```python
from build123d import *

# Parameters (mm, degrees)
SKETCH1_W           = 12.7
SKETCH1_H           = 9.525
BOSS_EXTRUDE1_DEPTH = 2.54
FILLET1_R           = 0.635
SHELL1_START        = 0.635
SHELL1_OUTLINE_W    = 1.905
SHELL1_OUTLINE_H    = 8.255
SHELL1_DEPTH        = 11.43
SKETCH2_R           = 2.54
BOSS_EXTRUDE2_DEPTH = 1.905
BOSS_EXTRUDE3_DEPTH = 0.00254


# Read off the part's stored shape, not the designer's step: Shell1
with BuildPart() as part:
    # Sketch1 → Boss-Extrude1 (new body)
    with BuildSketch(Plane(origin=(0, 0, 0), x_dir=(1, 0, 0), z_dir=(0, 1, 0))):
        with Locations((6.35, 4.7625)):
            Rectangle(SKETCH1_W, SKETCH1_H)
    extrude(amount=BOSS_EXTRUDE1_DEPTH)

    # Fillet1
    fillet1_edges = [part.edges().sort_by_distance(p)[0] for p in [
        (0, 1.27, -9.525),
        (12.7, 1.27, -9.525),
        (12.7, 1.27, 0),
        (0, 1.27, 0),
    ]]
    fillet(fillet1_edges, radius=FILLET1_R)

    # Shell1 outline → Shell1 (cut)
    with BuildSketch(Plane.YZ.offset(SHELL1_START)):
        with Locations((0.9525, -4.7625)):
            Rectangle(SHELL1_OUTLINE_W, SHELL1_OUTLINE_H)
    extrude(amount=SHELL1_DEPTH, mode=Mode.SUBTRACT)

    # Sketch2 → Boss-Extrude2 (add)
    with BuildSketch(Plane(origin=(0, 1.905, 0), x_dir=(-1, 0, 0), z_dir=(0, -1, 0))):
        with Locations(Location((-6.35, 4.7625, 0), (0, 0, 270))):
            Circle(SKETCH2_R)
    extrude(amount=BOSS_EXTRUDE2_DEPTH)

    # Sketch3 → Boss-Extrude3 (add)
    with BuildSketch(Plane(origin=(0, 2.54, 0), x_dir=(1, 0, 0), z_dir=(0, 1, 0))):
        Polygon((4.557346154, 6.477), (6.104141026, 6.477), (6.104141026, 5.907128205), (5.127217949, 5.907128205), (5.127217949, 5.296551282), (6.104141026, 5.296551282), (6.104141026, 4.726679487), (5.127217949, 4.726679487), (5.127217949, 3.302), (4.557346154, 3.302), align=None)
        with BuildLine():
            Line((7.162474359, 5.703602564), (6.592602564, 5.703602564))
            add(Edge.make_bspline(
                [(6.592602564, 5.703602564), (6.596626076, 5.732088422), (6.604513904, 5.78793306), (6.623388421, 5.868782184), (6.645964381, 5.945473111), (6.674149313, 6.017762976), (6.707205653, 6.085780553), (6.744797255, 6.149759244), (6.787330498, 6.20942444), (6.81993268, 6.245366991), (6.836197316, 6.263298077)],
                knots=[0, 0, 0, 0, 1.111473889, 2.178970933, 3.205615836, 4.199322666, 5.174200091, 6.12565194, 7.064921805, 8, 8, 8, 8], degree=3))
            add(Edge.make_bspline(
                [(6.836197316, 6.263298077), (6.859656898, 6.286956845), (6.905893269, 6.333585791), (6.983159668, 6.39331232), (7.064149124, 6.44500157), (7.150485915, 6.48598118), (7.240826576, 6.519149428), (7.335889528, 6.541428614), (7.435286308, 6.556211051), (7.503112106, 6.557667173), (7.53772476, 6.558410256)],
                knots=[0, 0, 0, 0, 1.01925491, 2.00884431, 2.983262333, 3.955970413, 4.92937149, 5.924503185, 6.940838805, 8, 8, 8, 8], degree=3))
            add(Edge.make_bspline(
                [(7.53772476, 6.558410256), (7.56849719, 6.55768378), (7.628989587, 6.556255673), (7.71789819, 6.544791605), (7.802665103, 6.524684907), (7.884186336, 6.49839585), (7.961262978, 6.462625195), (8.035596185, 6.421103078), (8.105109084, 6.370174475), (8.169964323, 6.31263028), (8.22954623, 6.2503906), (8.281144422, 6.1838615), (8.325504313, 6.114820126), (8.362050997, 6.042692875), (8.39015043, 5.9673577), (8.40965227, 5.8892498), (8.422416697, 5.808541527), (8.423688368, 5.753685202), (8.424333333, 5.725863181)],
                knots=[0, 0, 0, 0, 1.091422571, 2.145516843, 3.172569842, 4.178562979, 5.178154469, 6.181868002, 7.194278174, 8.227918432, 9.254613415, 10.245994977, 11.209837596, 12.161663635, 13.10878368, 14.055455738, 15.013766427, 16, 16, 16, 16], degree=3))
            add(Edge.make_bspline(
                [(8.424333333, 5.725863181), (8.423009825, 5.691407926), (8.420404245, 5.623576121), (8.399023573, 5.524299234), (8.365557006, 5.429372814), (8.317211295, 5.340125024), (8.256766844, 5.256798746), (8.182603526, 5.182179827), (8.096833706, 5.115098345), (8.032445159, 5.079048748), (7.999473558, 5.060588742)],
                knots=[0, 0, 0, 0, 0.992805628, 1.954529043, 2.915727527, 3.886831945, 4.871318353, 5.87440735, 6.911542536, 8, 8, 8, 8], degree=3))
            add(Edge.make_bspline(
                [(7.999473558, 5.060588742), (8.022104759, 5.053158442), (8.066574055, 5.038558236), (8.129781812, 5.009803295), (8.189885167, 4.978378911), (8.245849161, 4.94187206), (8.298230423, 4.901758919), (8.346709632, 4.857696584), (8.391576439, 4.809781133), (8.432098412, 4.757749048), (8.468063246, 4.702432482), (8.500332577, 4.645109215), (8.526892035, 4.584909929), (8.549391202, 4.52252214), (8.566520788, 4.45738514), (8.578581546, 4.389751328), (8.585552961, 4.319774984), (8.58661622, 4.272366053), (8.587153846, 4.248394231)],
                knots=[0, 0, 0, 0, 1.059543567, 2.081955587, 3.086750234, 4.076226789, 5.052108497, 6.020845489, 6.989030705, 7.970690546, 8.952259656, 9.923888338, 10.895517021, 11.877585046, 12.873342345, 13.889638361, 14.932918083, 16, 16, 16, 16], degree=3))
            add(Edge.make_bspline(
                [(8.587153846, 4.248394231), (8.586064006, 4.213165386), (8.583915064, 4.143701278), (8.570253093, 4.041387755), (8.544816966, 3.943840902), (8.511354332, 3.849938294), (8.46671881, 3.760892179), (8.414190304, 3.674659071), (8.349622216, 3.594229511), (8.277865874, 3.517477148), (8.198176272, 3.447697337), (8.111779779, 3.387201381), (8.020576181, 3.335285086), (7.923988457, 3.29313796), (7.822050165, 3.260679852), (7.714988515, 3.237217635), (7.602353665, 3.222863063), (7.525471567, 3.221358258), (7.486207332, 3.220589744)],
                knots=[0, 0, 0, 0, 1.005138573, 1.981928558, 2.936866704, 3.876260664, 4.820238198, 5.773547, 6.751179199, 7.756627054, 8.768222608, 9.766606018, 10.760583154, 11.757261445, 12.767156078, 13.807575856, 14.880313354, 16, 16, 16, 16], degree=3))
            add(Edge.make_bspline(
                [(7.486207332, 3.220589744), (7.449063998, 3.221400012), (7.376435124, 3.222984385), (7.270200196, 3.236697937), (7.169233952, 3.258819009), (7.073278726, 3.290000494), (6.98270576, 3.330437552), (6.896693704, 3.378589014), (6.816958908, 3.437232146), (6.742612971, 3.503719685), (6.67530511, 3.578314929), (6.615147733, 3.659289915), (6.56346732, 3.746952559), (6.52005193, 3.84092833), (6.485240973, 3.941382088), (6.457782192, 4.048109556), (6.438601784, 4.161319247), (6.432760351, 4.239209923), (6.429782051, 4.278923077)],
                knots=[0, 0, 0, 0, 1.066544725, 2.085487077, 3.070979577, 4.031932826, 4.977951092, 5.916076795, 6.857635327, 7.814973522, 8.776389752, 9.738577119, 10.707772778, 11.69409279, 12.707140348, 13.757286496, 14.856535458, 16, 16, 16, 16], degree=3))
            Line((6.429782051, 4.278923077), (6.999653846, 4.278923077))
            add(Edge.make_bspline(
                [(6.999653846, 4.278923077), (7.003265064, 4.258954782), (7.010298859, 4.220061291), (7.024017843, 4.163752162), (7.041895594, 4.111775358), (7.062566722, 4.063668911), (7.084894652, 4.018801199), (7.111872131, 3.978829299), (7.141522391, 3.942667809), (7.184307932, 3.899678631), (7.245472811, 3.855509046), (7.32806566, 3.817123574), (7.419942383, 3.794624972), (7.484173376, 3.791880212), (7.517372196, 3.790461538)],
                knots=[0, 0, 0, 0, 0.928156231, 1.807827665, 2.648129825, 3.438902246, 4.202261636, 4.936546065, 5.639352463, 6.338805438, 7.70633318, 9.064371875, 10.482673459, 12, 12, 12, 12], degree=3))
            add(Edge.make_bspline(
                [(7.517372196, 3.790461538), (7.534988663, 3.790763632), (7.569495381, 3.791355365), (7.620180613, 3.797913931), (7.668465432, 3.808715896), (7.714439772, 3.823395366), (7.758396309, 3.841796999), (7.799495209, 3.865524803), (7.83857417, 3.893111763), (7.875208368, 3.92412683), (7.909059122, 3.95792215), (7.937224941, 3.995344725), (7.96296646, 4.033372751), (7.982005074, 4.074494153), (7.998687001, 4.116496162), (8.008897192, 4.160903319), (8.01660662, 4.206784081), (8.017054661, 4.23818286), (8.017282051, 4.254118389)],
                knots=[0, 0, 0, 0, 1.110435564, 2.175094844, 3.216326037, 4.226890168, 5.215276772, 6.21526065, 7.213097102, 8.228249917, 9.239874822, 10.221364777, 11.178138315, 12.128914389, 13.072518965, 14.022636769, 14.996447288, 16, 16, 16, 16], degree=3))
            add(Edge.make_bspline(
                [(8.017282051, 4.254118389), (8.016678373, 4.271546606), (8.015476588, 4.306242192), (8.005657881, 4.356873103), (7.990152068, 4.40557596), (7.968612599, 4.452135082), (7.939849038, 4.496378862), (7.905908357, 4.539194964), (7.864116592, 4.578354886), (7.818265429, 4.617063282), (7.765096093, 4.65080533), (7.707198004, 4.681944282), (7.643049511, 4.706721274), (7.574216537, 4.728851717), (7.499397041, 4.74501545), (7.419055624, 4.756751894), (7.33332189, 4.765487859), (7.274224512, 4.766741177), (7.243884615, 4.767384615)],
                knots=[0, 0, 0, 0, 0.809814727, 1.612155564, 2.388397, 3.182215007, 3.988903953, 4.837162975, 5.715530372, 6.646997145, 7.623086902, 8.637258368, 9.698941581, 10.815059213, 11.996518529, 13.252603015, 14.589518788, 16, 16, 16, 16], degree=3))
            Line((7.243884615, 4.767384615), (7.243884615, 5.296551282))
            add(Edge.make_bspline(
                [(7.243884615, 5.296551282), (7.281659591, 5.29976832), (7.35232909, 5.30578676), (7.450422144, 5.319861093), (7.53300385, 5.338673756), (7.602059062, 5.361370215), (7.659398085, 5.390518382), (7.709489139, 5.422696672), (7.752629925, 5.460067052), (7.789089675, 5.501515143), (7.818256341, 5.546026507), (7.838898809, 5.592909304), (7.852530015, 5.640712924), (7.853821571, 5.673409158), (7.854461538, 5.689610176)],
                knots=[0, 0, 0, 0, 1.70044513, 3.18119609, 4.440695891, 5.496282586, 6.431922213, 7.318171381, 8.16090191, 8.983045123, 9.787564368, 10.536848927, 11.275007137, 12, 12, 12, 12], degree=3))
            add(Edge.make_bspline(
                [(7.854461538, 5.689610176), (7.853357412, 5.710280916), (7.85120239, 5.750625824), (7.834465326, 5.808367886), (7.805411679, 5.859840149), (7.766455839, 5.9049343), (7.718986794, 5.942600315), (7.663344752, 5.969945199), (7.600737148, 5.98601154), (7.556689325, 5.987677078), (7.533908654, 5.988538462)],
                knots=[0, 0, 0, 0, 1.009664648, 1.970651636, 2.907870547, 3.878035693, 4.867062054, 5.849714035, 6.887914197, 8, 8, 8, 8], degree=3))
            add(Edge.make_bspline(
                [(7.533908654, 5.988538462), (7.513260536, 5.987522119), (7.472288347, 5.985505385), (7.412374743, 5.970453015), (7.355476781, 5.945114223), (7.302772655, 5.910173522), (7.255023163, 5.868211222), (7.215834605, 5.818515587), (7.183239421, 5.764063969), (7.169423181, 5.723835374), (7.162474359, 5.703602564)],
                knots=[0, 0, 0, 0, 0.98818071, 1.960853194, 2.938124878, 3.957524365, 4.978590984, 5.968022688, 6.978025184, 8, 8, 8, 8], degree=3))
        make_face()
    extrude(amount=BOSS_EXTRUDE3_DEPTH)


solid = part.part
```
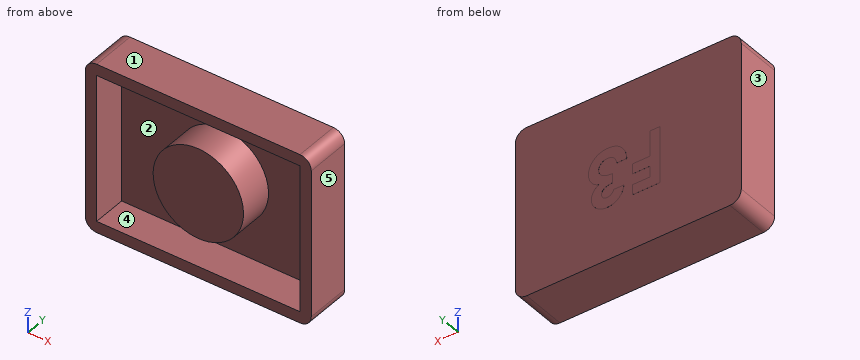
The listing builds one solid part. Answer for the finished solid, in the listing's coordinates (mm). Face numbers are marked on the shaded views. A direction names the side the tool comes from. Round coordinates to 2 decimals unless told otherwise and drop trailing zeros. Loops run counter-clockwise (first coordinate to the right, second up) from the corner with the lowest first, then second, coordinate; pieces in that order, holes last. Notation, with made-up numbers: (-25, 16) -> (23, 16) arc R29 ccw to (23, 37) -> close; hole circle Ø8 at (-25, 68.5). An arc over 180 degrees is marked (long way). Use one line per item in the form item = value.
1. The part is cut by section A-A on y = 1.7. Give the number of separate pieces and of enclosed holes in the cut face, and give its area (3 significant figures).
Answer key:
separate_pieces = 2
enclosed_holes = 1
area = 46.5 mm²
2. The part is cut by section C-C on x = 1. Determine the outline of the cut face in (y, z) (3 decimals), and give its area (3 significant figures).
Answer key:
outline = (0, -9.525) -> (2.54, -9.525) -> (2.54, 0) -> (0, 0) -> (0, -0.635) -> (1.905, -0.635) -> (1.905, -8.89) -> (0, -8.89) -> close
area = 8.47 mm²
3. A tool of negligible diameter and unlimited length cuts with its end or side. For the marked faces 4 and 5, from which of +Z, -Z, +X, -X, +Y, -Y can it reach the whole face along a straight path? Write none if from no direction.
Answer key:
face_4 = -Y
face_5 = +Z, -Z, +X, +Y, -Y
4. A flat-ended cylindrical pin translates along its axis: pin 1 Ø2.5 at (x, z) = (8, -4.5) entering from -Y. Find the tip coordinate at first contact, or state that the pin passes through.
Answer key:
pin_1 = 0
5. Find the intervals of material crossed by probe 1 along X at (y, z) = (0.7, -6.5) (3 decimals); probe 2 along X at (y, z) = (1.45, -8.75) (3 decimals); probe 3 along Z at (x, y) = (5.75, 1.5) (3 decimals), in increasing order. Write a range as [from, to].
Answer key:
probe_1 = [0, 0.635], [4.497, 8.203], [12.065, 12.7]
probe_2 = [0, 0.635], [12.065, 12.7]
probe_3 = [-9.525, -8.89], [-7.231, -2.294], [-0.635, 0]
6. The part is cut by section B-B on z = -1. Determine the outline of the cut face in (x, y) (3 decimals), and give its area (3 significant figures).
Answer key:
outline = (0, 0) -> (0.635, 0) -> (0.635, 1.905) -> (12.065, 1.905) -> (12.065, 0) -> (12.7, 0) -> (12.7, 2.54) -> (0, 2.54) -> close
area = 10.5 mm²
7. The part is cut by section D-D on x = 4. Determine the outline of the cut face in (y, z) (3 decimals).
Answer key:
outline = (0, -9.525) -> (2.54, -9.525) -> (2.54, 0) -> (0, 0) -> (0, -0.635) -> (1.905, -0.635) -> (1.905, -3.799) -> (0, -3.799) -> (0, -5.726) -> (1.905, -5.726) -> (1.905, -8.89) -> (0, -8.89) -> close
8. For a pull along X with two mould halves and no side action, classify the marked faces 1, 2 and 3 as released by +X, released by -X, zero draft, split by the parting line, or undercut.
Answer key:
face_1 = zero draft
face_2 = undercut
face_3 = released by -X
